```python
from build123d import *

# Parameters (mm, degrees)
F0_W     = 30
F0_H     = 20
F1_DEPTH = 1.5
F2_W     = 30
F2_H     = 2
F3_DEPTH = 3
F4_W     = 10
F4_H     = 5
F5_DEPTH = 10
F6_W     = 7.152542
F6_H     = 10
F7_DEPTH = 8


with BuildPart() as f1:
    # F0 (on Top) → F1 (new body)
    with BuildSketch(Plane.XY):
        Rectangle(F0_W, F0_H)
    extrude(amount=F1_DEPTH)

    # F2 (on face) → F3 (join)
    with BuildSketch(Plane.XY.offset(1.5)):
        with Locations((0, 7.468739)):
            Rectangle(F2_W, F2_H)
    extrude(amount=F3_DEPTH)

    # F4 (on face) → F5 (join)
    with BuildSketch(Plane(origin=(0, 0, 0), x_dir=(1, 0, 0), z_dir=(0, 0, -1))):
        with Locations((0, 2.5)):
            Rectangle(F4_W, F4_H)
        with Locations((0, -2.5)):
            Rectangle(F4_W, F4_H)
    extrude(amount=F5_DEPTH)

    # F6 (on face) → F7 (cut)
    with BuildSketch(Plane(origin=(0, 0, -10), x_dir=(1, 0, 0), z_dir=(0, 0, -1))):
        Rectangle(F6_W, F6_H)
    extrude(amount=-F7_DEPTH, mode=Mode.SUBTRACT)


solid = f1.part
```
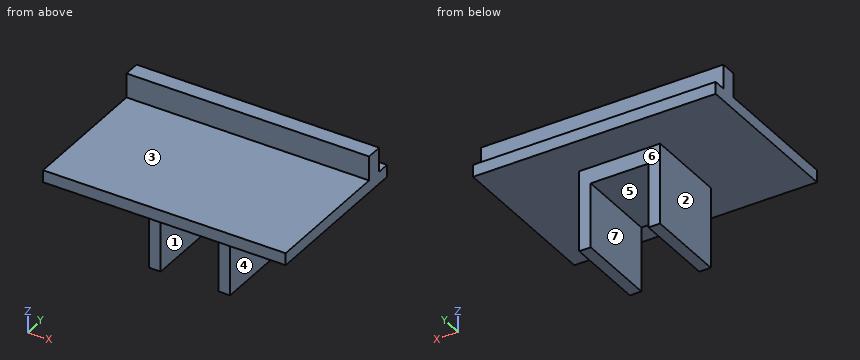
Source: CAD feature listing. Evaluate the final solid. Frame: model axes, mm. Face numbers are marked on the shaded views. A direction names the side the tool comes from. Round coordinates to 2 decimals unless told otherwise and drop trailing zeros. Loops run counter-clockwise (first coordinate to the right, second up) from the corner with the lowest first, then second, coordinate; pieces in that order, holes last.
1. Section query D-D on x = 11.5. Output: boundary loops of the cut face in (y, z), and give its area (3 significant figures).
2. Ray query, L1, parallel to X at y = 2.5, z = -9.5; L2, parallel to Z at x = 8.5, y = -7; L3, parallel to Y at x = -4.75, z = 3. Return the intervals inside material, ascending.
3. Section query B-B on y = -0.25. Output: boundary loops of the cut face in (x, z), and give its area (3 significant figures).
4. Mould query, pull axis X, two halves, no side actions, for the marked faces 4, 5, 6 and 7. Classes: released by +X, released by -X, zero draft, split by the parting line, or undercut.
5. Section query A-A on z = -6. Output: boundary loops of the cut face in (x, y), and give its area (3 significant figures).
6. Contact query for flat-ended pins moving along their axis: pin 1 (3.5 mm diameter, centred on x = 6, z = 3, fed in from -Y); pin 2 (8 mm diameter, centred on y = -1.5, z = -7.5, fed in from -X); pin 3 (1.5 mm diameter, centred on x = 4.5, z = -4, fed in from +Y); pin 4 (0.5 mm diameter, centred on x = -6, y = 9.5, fed in from +Z). Output: stop coordinate, or through.
7. Access query for the marked faces 1, 2 and 3. Directions: +Z, -Z, +X, -X, +Y, -Y. A direction counts if a zero-diameter tool reaches every point of the face in a straight line with its end or side. Return the directions, or none.
8. Section query C-C on x = 4.25. Output: boundary loops of the cut face in (y, z).
Answers below:
1. outline: (-10, 0) - (10, 0) - (10, 1.5) - (8.47, 1.5) - (8.47, 4.5) - (6.47, 4.5) - (6.47, 1.5) - (-10, 1.5) - close
1. area: 36.0 mm2
2. L1: x = -5 to -3.58, 3.58 to 5
2. L2: z = 0 to 1.5
2. L3: y = 6.47 to 8.47
3. outline: (-15, 0) - (-5, 0) - (-5, -10) - (-3.58, -10) - (-3.58, -2) - (3.58, -2) - (3.58, -10) - (5, -10) - (5, 0) - (15, 0) - (15, 1.5) - (-15, 1.5) - close
3. area: 87.8 mm2
4. face 4: released by +X
4. face 5: undercut
4. face 6: zero draft
4. face 7: undercut
5. outline: (-5, -5) - (-3.58, -5) - (-3.58, 5) - (-5, 5) - close; (3.58, -5) - (5, -5) - (5, 5) - (3.58, 5) - close
5. area: 28.5 mm2
6. pin 1: stops at y = -10
6. pin 2: stops at x = -5
6. pin 3: stops at y = 5
6. pin 4: stops at z = 1.5
7. face 1: -Z, +Y, -Y
7. face 2: -Z, -X, +Y, -Y
7. face 3: +Z, +X, -X, -Y
8. outline: (-10, 0) - (-5, 0) - (-5, -10) - (5, -10) - (5, 0) - (10, 0) - (10, 1.5) - (8.47, 1.5) - (8.47, 4.5) - (6.47, 4.5) - (6.47, 1.5) - (-10, 1.5) - close
